from build123d import *

# Parameters (mm, degrees)
SKETCH_1_R      = 1.499696603
SKETCH_1_R_2    = 0.75
EXTRUDE_1_DEPTH = 3


with BuildPart() as part:
    # 草图1 → 凸台-拉伸1 (new body)
    with BuildSketch(Plane.XY):
        Polygon((0, 0), (0, -18), (1.5, -18), (1.5, -15), (4.5, -15), (4.5, -18), (34.5, -18), (34.5, -14), (37.5, -14), (37.5, -18), (67.5, -18), (67.5, -15), (70.5, -15), (70.5, -18), (72, -18), (72, 0), (70.5, 0), (70.5, -3), (67.5, -3), (67.5, 0), (37.5, 0), (37.5, -4), (34.5, -4), (34.5, 0), (4.5, 0), (4.5, -3), (1.5, -3), (1.5, 0), align=None)
        with Locations((36, -9)):
            Circle(SKETCH_1_R, mode=Mode.SUBTRACT)
        with Locations((31.683762096, -9)):
            Circle(SKETCH_1_R_2, mode=Mode.SUBTRACT)
        with Locations((4.183762096, -9)):
            Circle(SKETCH_1_R_2, mode=Mode.SUBTRACT)
        with Locations(Location((67.816237904, -9, 0), (0, 0, 180))):
            Circle(SKETCH_1_R_2, mode=Mode.SUBTRACT)
        with Locations(Location((40.316237904, -9, 0), (0, 0, 180))):
            Circle(SKETCH_1_R_2, mode=Mode.SUBTRACT)
        Polygon((29.5, -9), (29.5, -15), (6.5, -15), (6.5, -3), (29.5, -3), align=None, mode=Mode.SUBTRACT)
        Polygon((42.5, -3), (42.5, -9), (42.5, -15), (65.5, -15), (65.5, -3), align=None, mode=Mode.SUBTRACT)
    extrude(amount=EXTRUDE_1_DEPTH)


solid = part.part
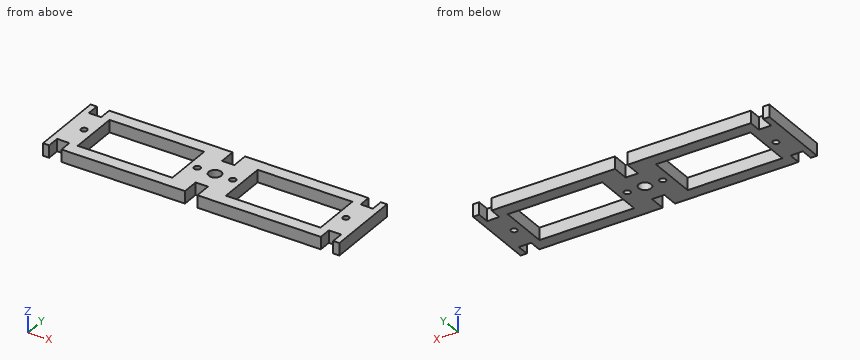
Here's how the part is built. I have some questions about the finished solid (model axes, mm). Coordinates: 2 decimals unless noted, no trailing zeros. Write each loop counter-clockwise with the first axis right and the second up, starting at its lowest first coordinate (ties: lowest second). Pieces come first, ordered by that corner, then holes.
1) If we section it at B-B (x = 14.5): List the corners of the cut face in (y, z) for me.
Filled in:
outline: (-18, 0) - (-15, 0) - (-15, 3) - (-18, 3) - close; (-3, 0) - (0, 0) - (0, 3) - (-3, 3) - close
2) If we section it at C-C (y = -9): Count the separate pieces of the cut face and the enclosed holes in it, plus the area to 3 significant figures.
Filled in:
separate pieces: 8
enclosed holes: 0
area: 51.0 mm2
3) I'm going to push flat-ended pins straight in: pin 1 (10 mm diameter, centred on x = 38, y = -11, fed in from -Z); pin 2 (1.5 mm diameter, centred on x = 36, z = 1.5, fed in from +Y). Where does each tip first touch, or does it pass through?
Filled in:
pin 1: stops at z = 0
pin 2: stops at y = -4
4) If I drill on line 1 (X direction, y = -16.75, z = 0.75); line 2 (X direction, y = -12.25, z = 0.75); line 3 (Y direction, x = 12, z = 1.45), over which ranges is the centre line in solid material (lowest first)?
Filled in:
line 1: x = 0 to 1.5, 4.5 to 34.5, 37.5 to 67.5, 70.5 to 72
line 2: x = 0 to 6.5, 29.5 to 42.5, 65.5 to 72
line 3: y = -18 to -15, -3 to 0
5) If we section it at A-A (y = -11.75): List the corners of the cut face in (x, z) for me, plus the area to 3 significant figures.
Filled in:
outline: (0, 0) - (6.5, 0) - (6.5, 3) - (0, 3) - close; (29.5, 0) - (42.5, 0) - (42.5, 3) - (29.5, 3) - close; (65.5, 0) - (72, 0) - (72, 3) - (65.5, 3) - close
area: 78.0 mm2
6) If we section it at D-D (y = -16.5): List the corners of the cut face in (x, z) for me.
Filled in:
outline: (0, 0) - (1.5, 0) - (1.5, 3) - (0, 3) - close; (4.5, 0) - (34.5, 0) - (34.5, 3) - (4.5, 3) - close; (37.5, 0) - (67.5, 0) - (67.5, 3) - (37.5, 3) - close; (70.5, 0) - (72, 0) - (72, 3) - (70.5, 3) - close
